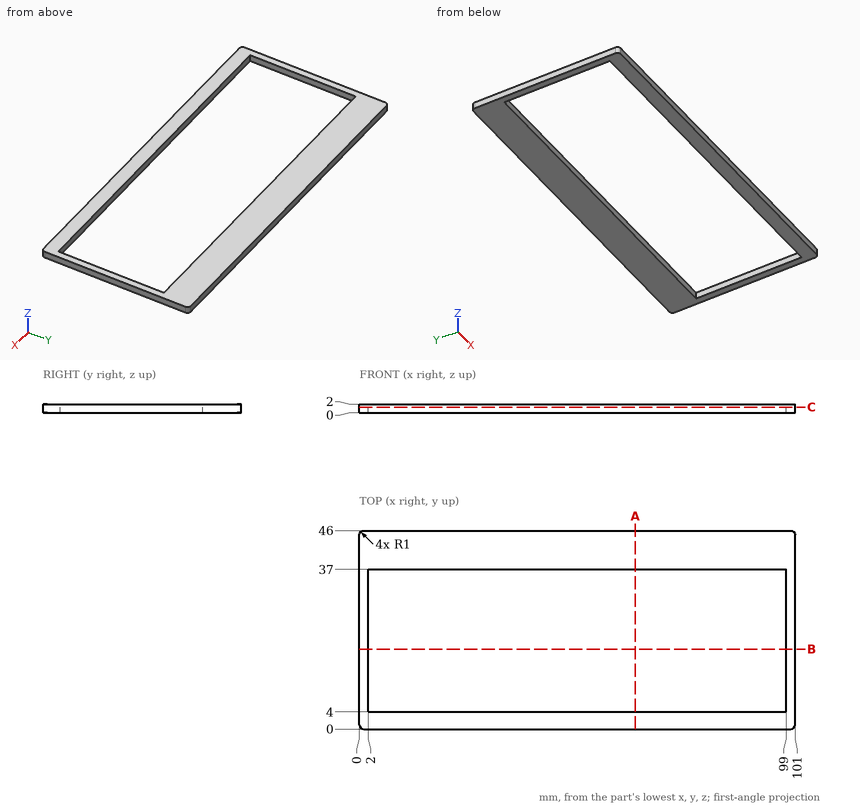
Could you check a few things on this drawing? It's one solid part, dimensions in mm from its lowest x, y, z. Give positions to 0.01 mm unless a question says otherwise; leave off trailing zeros. Order: outer loops, then holes, each group sorted by start corner. A loop starts at its lowest first (then second) coordinate and runs counter-clockwise, first axis right, second up. Notation, with made-up numbers: M 7,30.25 L 36,30.25 A10 cw 36,46.25 Z; hole C 13,83.5 d5. An arc over 180 degrees is marked long. Use one line per item in the form item = value.
Item 1: If we section it at A-A, the plane x = 64: Write out the boundary of the cut face in (y, z).
Values follow:
outline = M 0,0 L 4,0 L 4,2 L 0,2 Z; M 37,0 L 46,0 L 46,2 L 37,2 Z
Item 2: If I drill on line 1 along Y through (x, z) = (68, 1.05); line 2 along X through (y, z) = (9, 1.1), over which ranges is the centre line in solid material (lowest first)? Write a range as [from, to].
Values follow:
line_1 = [0, 4], [37, 46]
line_2 = [0, 2], [99, 101]
Item 3: If we section it at B-B, the plane y = 18.5: Write out the boundary of the cut face in (x, z).
Values follow:
outline = M 0,0 L 2,0 L 2,2 L 0,2 Z; M 99,0 L 101,0 L 101,2 L 99,2 Z
Item 4: If we section it at C-C, the plane z = 1.25: Write out the boundary of the cut face in (x, y).
Values follow:
outline = M 0,1 A1 ccw 1,0 L 100,0 A1 ccw 101,1 L 101,45 A1 ccw 100,46 L 1,46 A1 ccw 0,45 Z; hole M 2,4 L 99,4 L 99,37 L 2,37 Z
